from build123d import *

# Parameters (mm, degrees)
F0_R     = 2.54
F1_DEPTH = 2.032


with BuildPart() as f1:
    # F0 (on Top) → F1 (new body)
    with BuildSketch(Plane.XY):
        with BuildLine():
            ThreePointArc((19.05, -77.704174), (23.540128, -75.844302), (25.4, -71.354174))
            Line((25.4, -71.354174), (25.4, 42.945826))
            ThreePointArc((25.4, 42.945826), (23.540128, 47.435954), (19.05, 49.295826))
            Line((19.05, 49.295826), (6.35, 49.295826))
            ThreePointArc((6.35, 49.295826), (1.859872, 47.435954), (0, 42.945826))
            Line((0, 42.945826), (0, 26.526082))
            ThreePointArc((0, 26.526082), (-0.483365, 24.096043), (-1.859872, 22.035954))
            Line((-1.859872, 22.035954), (-23.540128, 0.355698))
            ThreePointArc((-23.540128, 0.355698), (-25.600216, -1.020809), (-28.030256, -1.504174))
            Line((-28.030256, -1.504174), (-44.45, -1.504174))
            ThreePointArc((-44.45, -1.504174), (-48.940128, -3.364046), (-50.8, -7.854174))
            Line((-50.8, -7.854174), (-50.8, -14.204174))
            Line((-50.8, -14.204174), (-50.8, -20.554174))
            ThreePointArc((-50.8, -20.554174), (-48.940128, -25.044302), (-44.45, -26.904174))
            Line((-44.45, -26.904174), (-28.030256, -26.904174))
            ThreePointArc((-28.030256, -26.904174), (-25.600216, -27.387539), (-23.540128, -28.764046))
            Line((-23.540128, -28.764046), (-1.859872, -50.444302))
            ThreePointArc((-1.859872, -50.444302), (-0.483365, -52.50439), (0, -54.93443))
            Line((0, -54.93443), (0, -71.354174))
            ThreePointArc((0, -71.354174), (1.859872, -75.844302), (6.35, -77.704174))
            Line((6.35, -77.704174), (12.7, -77.704174))
            Line((12.7, -77.704174), (19.05, -77.704174))
        make_face()
        with BuildLine():
            ThreePointArc((15.24, -65.004174), (14.496051, -66.800225), (12.7, -67.544174))
            ThreePointArc((12.7, -67.544174), (10.903949, -63.208123), (15.24, -65.004174))
        make_face(mode=Mode.SUBTRACT)
        with Locations((0, -23.729174)):
            Circle(F0_R, mode=Mode.SUBTRACT)
        with Locations((12.7, -39.604174)):
            Circle(F0_R, mode=Mode.SUBTRACT)
        with Locations((-38.1, -14.204174)):
            Circle(F0_R, mode=Mode.SUBTRACT)
        with Locations((-12.7, -14.204174)):
            Circle(F0_R, mode=Mode.SUBTRACT)
        with Locations((0, -4.679174)):
            Circle(F0_R, mode=Mode.SUBTRACT)
        with Locations((12.7, -14.204174)):
            Circle(F0_R, mode=Mode.SUBTRACT)
        with Locations((12.7, 11.195826)):
            Circle(F0_R, mode=Mode.SUBTRACT)
        with Locations((12.7, 36.595826)):
            Circle(F0_R, mode=Mode.SUBTRACT)
    extrude(amount=F1_DEPTH)


solid = f1.part
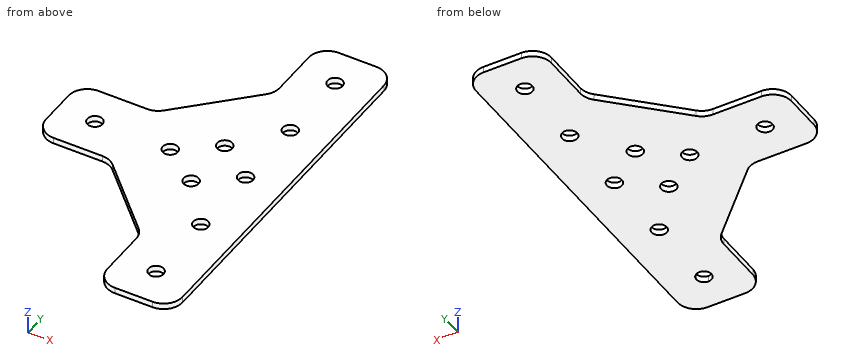
Input: part model. Units: mm. Frame: model coordinates. Round coordinates to 2 decimals unless told otherwise and drop trailing zeros. Loops run counter-clockwise (first coordinate to the right, second up) from the corner with the lowest first, then second, coordinate; pieces in that order, holes last. Notation, with made-up numbers: M -26,-38.5 L 22,-38.5 A19 ccw 22,-5.5 Z; hole C 48.25,24.25 d8. An arc over 180 degrees is marked long. Answer as CSV lines item,"result". Start each with the question number.
(1) Section D-D, the plane x = -29.5. Output: boundary loops of the cut face in (y, z), plus the area to 3 significant figures.
(2) Section A-A, the plane x = -38.1. Output: boundary loops of the cut face in (y, z), plus the area to 3 significant figures.
(3) Line query: line 1 (Y direction, x = 12.5, z = 1.4); line 2 (Y direction, x = -38, z = 1.3); line 3 (Y direction, x = 11.5, z = 1). Output: solid intervals per line, ascending. Write a range as [from, to].
(4) Section B-B, the plane z = 1.5. State how many separate pieces and enclosed holes the cut face has, plus the area to 3 significant figures.
(5) First-contact query: pin 1 (4.5 mm diameter, centred on x = 12.7, y = 36.6, fed in from +Z); pin 2 (0.6 mm diameter, centred on x = -39, z = 0.5, fed in from +Y). Flat tips, straight axial feed; report the tip coordinate or a pass-through.
(6) Section C-C, the plane y = 28. Output: boundary loops of the cut face in (x, z), plus the area to 3 significant figures.
Values found:
1,outline,"M -26.9,0 L -1.5,0 L -1.5,2.03 L -26.9,2.03 Z"
1,area,"51.6 mm²"
2,outline,"M -26.9,0 L -16.74,0 L -16.74,2.03 L -26.9,2.03 Z; M -11.66,0 L -1.5,0 L -1.5,2.03 L -11.66,2.03 Z"
2,area,"41.3 mm²"
3,line 1,"y = [-77.7, -67.54], [-62.47, -42.14], [-37.07, -16.74], [-11.67, 8.66], [13.73, 34.06], [39.13, 49.3]"
3,line 2,"y = [-26.9, -16.74], [-11.67, -1.5]"
3,line 3,"y = [-77.7, -67.24], [-62.77, -41.84], [-37.37, -16.44], [-11.97, 8.96], [13.43, 34.36], [38.83, 49.3]"
4,separate pieces,"1"
4,enclosed holes,"9"
4,area,"4,930 mm²"
5,pin 1,"passes through"
5,pin 2,"stops at y = -1.5"
6,outline,"M 0,0 L 25.4,0 L 25.4,2.03 L 0,2.03 Z"
6,area,"51.6 mm²"
